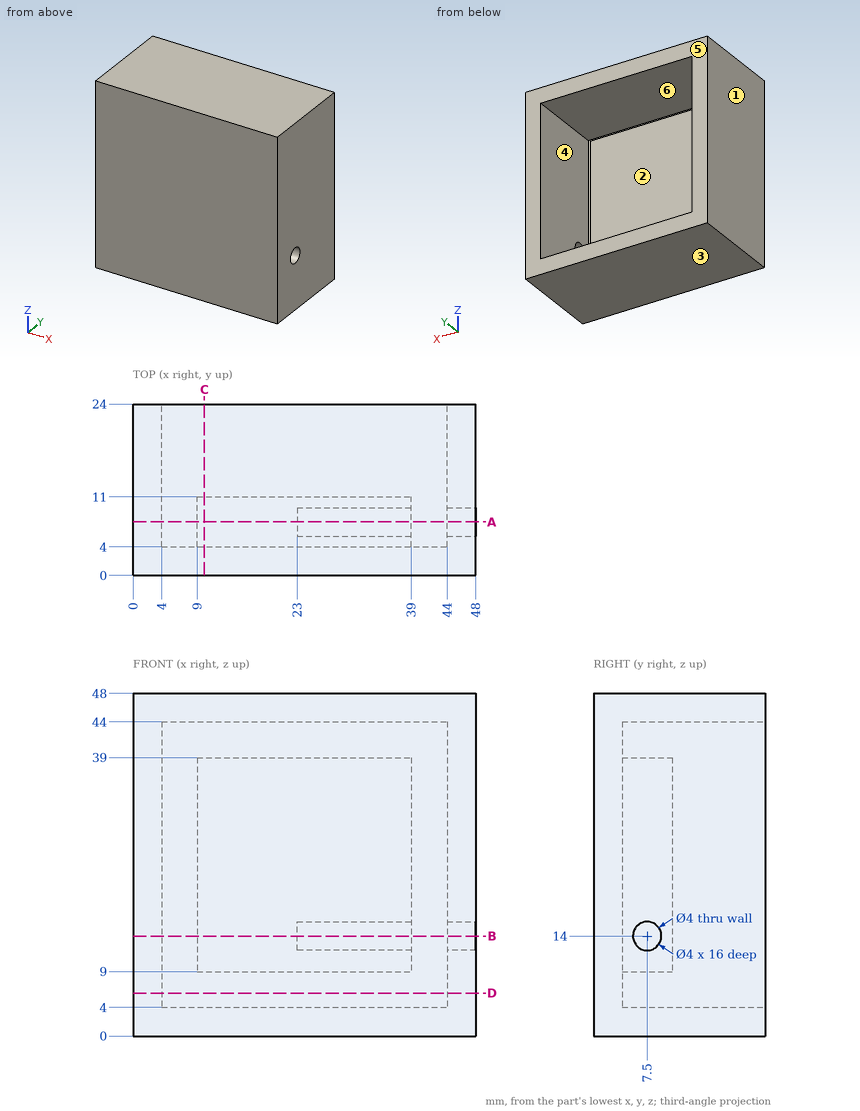
For this review, use the dimensioned drawing (mm, ordinates from the lowest corner) and the shaded views. A direction names the side the tool comes from. Round coordinates to 2 decimals unless told otherwise and drop trailing zeros. Order: outer loops, then holes, each group sorted by start corner. A loop starts at its lowest first (then second) coordinate and runs counter-clockwise, first axis right, second up. Notation, with made-up numbers: M 86.5,25.5 L 105.5,25.5 A15 ccw 105.5,47.5 Z; hole C -20.5,-15.5 d2. An arc over 180 degrees is marked long. Use a Markdown table: item, result. Add a question column.
Item 1: To check wall thickness, follow line 1 along Z through (x, y) = (15.5, 5.75); line 2 along X through (y, z) = (19.75, 26.5). State the ranges of each line that lie inside material, in increasing order.
Item 2: Insertion check: pin 1 (2 mm diameter, centred on y = 8, z = 14, fed in from +X); pin 2 (15 mm diameter, centred on x = 29.5, z = 21.5, fed in from +Y). Each pin has a flat end and moves straight along its axis. Give the tip position at first contact, or say it passes through.
Item 3: Add section A-A, the plane y = 7.5. Give the boundary of the cut face in (x, z), then the cut area to 3 significant figures.
Item 4: Add section D-D, the plane z = 6. Give the boundary of the cut face in (x, y), then the cut area to 3 significant figures.
Item 5: Tool access review of the marked faces 5 and 6: name each direction out of +Z, -Z, +X, -X, +Y, -Y from which nothing blocks a thin tool from reaching the whole face with its end or side.
Item 6: Add section C-C, the plane x = 10. Give the boundary of the cut face in (y, z).
Item 7: Mouldability with a two-part tool opening along Z and no side actions: class the marked faces 1, 2, 3 and 4 as released by +Z, released by -Z, zero draft, split by the parting line, or undercut.
Item 8: Add section B-B, the plane z = 14. Give the boundary of the cut face in (x, y), then the cut area to 3 significant figures.
Geometry results:
| question | item | result |
|---|---|---|
| 1 | line 1 | z = 0 to 4, 9 to 39, 44 to 48 |
| 1 | line 2 | x = 0 to 4, 44 to 48 |
| 2 | pin 1 | stops at x = 23 |
| 2 | pin 2 | stops at y = 11 |
| 3 | outline | M 0,0 L 48,0 L 48,12 L 44,12 L 44,4 L 4,4 L 4,44 L 44,44 L 44,16 L 48,16 L 48,48 L 0,48 Z; M 9,9 L 39,9 L 39,12 L 23,12 L 23,16 L 39,16 L 39,39 L 9,39 Z |
| 3 | area | 1,520 mm² |
| 4 | outline | M 0,0 L 48,0 L 48,24 L 44,24 L 44,4 L 4,4 L 4,24 L 0,24 Z |
| 4 | area | 352 mm² |
| 5 | face 5 | +Z, -Z, +X, -X, +Y |
| 5 | face 6 | +Y |
| 6 | outline | M 0,0 L 24,0 L 24,4 L 4,4 L 4,9 L 11,9 L 11,39 L 4,39 L 4,44 L 24,44 L 24,48 L 0,48 Z |
| 7 | face 1 | zero draft |
| 7 | face 2 | undercut |
| 7 | face 3 | released by -Z |
| 7 | face 4 | undercut |
| 8 | outline | M 0,0 L 48,0 L 48,5.5 L 44,5.5 L 44,4 L 39,4 L 39,5.5 L 23,5.5 L 23,9.5 L 39,9.5 L 39,11 L 9,11 L 9,4 L 4,4 L 4,24 L 0,24 Z; M 44,9.5 L 48,9.5 L 48,24 L 44,24 Z |
| 8 | area | 482 mm² |
